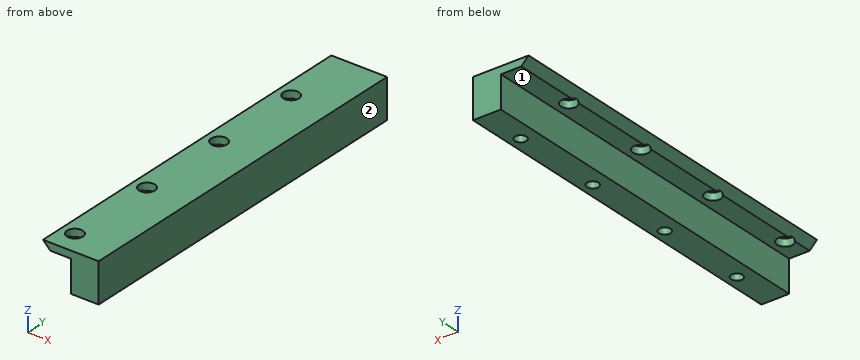
Autodesk Inventor part; units mm, degrees
ref_plane "Left_Connecting_Web_StartPlane" through (0, 0, 4) normal (0, 0, 1) x (1, 0, 0)
ref_plane "Left_Rod_Contact_Flange_StartPlane" through (0, 0, 10.9) normal (0, 0, 1) x (1, 0, 0)
ref_plane "Work Plane3" through (0, 0, 4) normal (0, 0, 1) x (1, 0, 0)
ref_plane "Left_Connecting_Web_StartPlane" through (0, 0, 4) normal (0, 0, 1) x (1, 0, 0)
sketch "Left_Connecting_Web_Profile" plane through (0, 0, 4) normal (0, 0, 1) x (1, 0, 0)
  line L0 (6, 0) -> (12, 0)
  line L1 (12, 0) -> (12, 80)
  line L2 (12, 80) -> (6, 80)
  line L3 (6, 80) -> (6, 0)
  point P0 (0, 0)
  dimension "d1" = 6
  dimension "d2" = 6
  dimension "d3" = 80
extrude "Left_Connecting_Web" add sketch "Left_Connecting_Web_Profile" along normal blind 8.5
ref_plane "Left_Rod_Contact_Flange_StartPlane" through (0, 0, 10.9) normal (0, 0, 1) x (1, 0, 0)
sketch "Left_Rod_Contact_Flange_Profile" plane through (0, 0, 10.9) normal (0, 0, 1) x (1, 0, 0)
  line L0 (0, 0) -> (12, 0)
  line L1 (12, 0) -> (12, 80)
  line L2 (12, 80) -> (0, 80)
  line L3 (0, 80) -> (0, 0)
  dimension "d7" = 12
  dimension "d8" = 80
extrude "Left_Rod_Contact_Flange" add sketch "Left_Rod_Contact_Flange_Profile" along normal blind 1.6
sketch "Original_Rod_Clearance_4x_Locations" plane through (0, 0, 0) normal (0, 0, 1) x (1, 0, 0)
  circle A0 centre (3, 5) radius 1.7
  circle A1 centre (3, 25) radius 1.7
  circle A2 centre (3, 45) radius 1.7
  circle A3 centre (3, 65) radius 1.7
  point P0 (0, 0)
  dimension "d11" = 3
  dimension "d12" = 5
  dimension "d13" = 3.4
  dimension "d14" = 3
  dimension "d15" = 25
  dimension "d16" = 3.4
  dimension "d17" = 3
  dimension "d18" = 45
  dimension "d19" = 3.4
  dimension "d20" = 3
  dimension "d21" = 65
  dimension "d22" = 3.4
extrude "Original_Rod_Clearance_4x" cut sketch "Original_Rod_Clearance_4x_Locations" along normal through all
ref_plane "Work Plane3" through (0, 0, 4) normal (0, 0, 1) x (1, 0, 0)
sketch "Deck_Assembly_M3_Locations" plane through (0, 0, 4) normal (0, 0, 1) x (1, 0, 0)
  circle A0 centre (9.5, 10) radius 1.25
  circle A1 centre (9.5, 30) radius 1.25
  circle A2 centre (9.5, 50) radius 1.25
  circle A3 centre (9.5, 70) radius 1.25
  point P0 (0, 0)
  dimension "d26" = 9.5
  dimension "d27" = 10
  dimension "d28" = 2.5
  dimension "d29" = 9.5
  dimension "d30" = 30
  dimension "d31" = 2.5
  dimension "d32" = 9.5
  dimension "d33" = 50
  dimension "d34" = 2.5
  dimension "d35" = 9.5
  dimension "d36" = 70
  dimension "d37" = 2.5
extrude "Four_Blind_M3_Tap_Bores" cut sketch "Deck_Assembly_M3_Locations" along normal blind 6.5
thread "Deck_M3x0_5_6H_1"
thread "Deck_M3x0_5_6H_2"
thread "Deck_M3x0_5_6H_3"
thread "Deck_M3x0_5_6H_4"
chamfer "Outer_End_1p6mm_45deg" distance 1.6 angle 45 1 edges at (0, 40, 10.9)
equation "\"d2\" = WebThickness"
equation "\"d3\" = ContactLength"
equation "\"d4\" = DropHeight"
equation "\"d7\" = RodWidth + WebThickness"
equation "\"d8\" = ContactLength"
equation "\"d9\" = RodFlangeThickness"
equation "\"d13\" = RodClearanceDiameter"
equation "\"d16\" = RodClearanceDiameter"
equation "\"d19\" = RodClearanceDiameter"
equation "\"d22\" = RodClearanceDiameter"
equation "\"d28\" = TapDrillDiameter"
equation "\"d31\" = TapDrillDiameter"
equation "\"d34\" = TapDrillDiameter"
equation "\"d37\" = TapDrillDiameter"
equation "\"d38\" = JoinThreadDepth"
equation "\"d40\" = JoinThreadDepth"
equation "\"d42\" = JoinThreadDepth"
equation "\"d44\" = JoinThreadDepth"
equation "\"d46\" = JoinThreadDepth"
equation "\"d48\" = OuterEndChamfer"
equation "\"d49\" = OuterEndChamfer"
equation "\"OverallWidth\" = 51"
equation "\"RodWidth\" = 6"
equation "\"ContactLength\" = 80"
equation "\"BaseThickness\" = 4"
equation "\"DropHeight\" = 8.5"
equation "\"WebThickness\" = 6"
equation "\"FingerStartX\" = 19.93338"
equation "\"FingerWidth\" = 13.5"
equation "\"FingerThickness\" = 6"
equation "\"FingerEndInset\" = 4"
equation "\"RodClearanceDiameter\" = 3.4"
equation "\"ClampFirstY\" = 41.82802"
equation "\"ClampPitch\" = 16"
equation "\"ClampHeight\" = BaseThickness + 0.5 * FingerThickness"
equation "\"TapDrillDiameter\" = 2.5"
equation "\"TapDepth\" = 6"
equation "\"RodHoleStart\" = 5"
equation "\"RodScrewPitch\" = 20"
equation "\"JoinLeftX\" = 9.5"
equation "\"JoinFirstY\" = 10"
equation "\"JoinPitch\" = 20"
equation "\"JoinThreadDepth\" = 6.5"
equation "\"JoinCountersinkDiameter\" = 6.2"
equation "\"d0\" = BaseThickness"
equation "\"d6\" = BaseThickness + DropHeight - RodFlangeThickness"
equation "\"d25\" = BaseThickness"
equation "\"RodFlangeThickness\" = 1.6"
equation "\"OuterEndChamfer\" = RodFlangeThickness"
properties part number "Left_Rod_Support"
Check sheet for the modelled part. Datum: model origin and axes. Units: mm. Face numbers are marked on the shaded views. A direction names the side the tool comes from. Round coordinates to 2 decimals unless told otherwise and drop trailing zeros. Loops run counter-clockwise (first coordinate to the right, second up) from the corner with the lowest first, then second, coordinate; pieces in that order, holes last. Notation, with made-up numbers: (62, 62.5) -> (109, 62.5) arc R33 ccw to (109, 96.5) -> close; hole circle Ø5 at (6, 15). An arc over 180 degrees is marked (long way). Answer in a Markdown table with one row per item.
Q1. Sectioned sample at D-D on x = 9.5. Enter the section's corners in (y, z).
Data:
| item | result |
|---|---|
| outline | (0, 4) -> (8.75, 4) -> (8.75, 10.5) -> (11.25, 10.5) -> (11.25, 4) -> (28.75, 4) -> (28.75, 10.5) -> (31.25, 10.5) -> (31.25, 4) -> (48.75, 4) -> (48.75, 10.5) -> (51.25, 10.5) -> (51.25, 4) -> (68.75, 4) -> (68.75, 10.5) -> (71.25, 10.5) -> (71.25, 4) -> (80, 4) -> (80, 12.5) -> (0, 12.5) -> close |
Q2. Set-up check for the marked faces 1 and 2: record each of +Z, -Z, +X, -X, +Y, -Y from which the full face is reachable in a straight line by a thin tool's end or side.
Data:
| item | result |
|---|---|
| face 1 | -Z, -X, +Y, -Y |
| face 2 | +Z, -Z, +X, +Y, -Y |
Q3. Thickness scan on L1, parallel to Y at x = 9.5, z = 5.75; L2, parallel to Y at x = 3, z = 11.6; L3, parallel to X at y = 19, z = 8.25. Record the ranges inside material, lowest first.
Data:
| item | result |
|---|---|
| L1 | y = 0 to 8.75, 11.25 to 28.75, 31.25 to 48.75, 51.25 to 68.75, 71.25 to 80 |
| L2 | y = 0 to 3.3, 6.7 to 23.3, 26.7 to 43.3, 46.7 to 63.3, 66.7 to 80 |
| L3 | x = 6 to 12 |
Q4. Sectioned sample at B-B on z = 5.25. Enter the section's corners in (x, y), then the cut area to 3 significant figures.
Data:
| item | result |
|---|---|
| outline | (6, 0) -> (12, 0) -> (12, 80) -> (6, 80) -> close; hole circle Ø2.5 at (9.5, 10); hole circle Ø2.5 at (9.5, 30); hole circle Ø2.5 at (9.5, 50); hole circle Ø2.5 at (9.5, 70) |
| area | 460 mm^2 |
Q5. Sectioned sample at A-A on y = 65. Enter the section's corners in (x, z), then the cut area to 3 significant figures.
Data:
| item | result |
|---|---|
| outline | (0, 12.5) -> (1.3, 11.2) -> (1.3, 12.5) -> close; (4.7, 10.9) -> (6, 10.9) -> (6, 4) -> (12, 4) -> (12, 12.5) -> (4.7, 12.5) -> close |
| area | 53.9 mm^2 |
Q6. Sectioned sample at C-C on y = 30. Enter the section's corners in (x, z), then the cut area to 3 significant figures.
Data:
| item | result |
|---|---|
| outline | (0, 12.5) -> (1.6, 10.9) -> (6, 10.9) -> (6, 4) -> (8.25, 4) -> (8.25, 10.5) -> (10.75, 10.5) -> (10.75, 4) -> (12, 4) -> (12, 12.5) -> close |
| area | 43.1 mm^2 |
Q7. Go/stop test with flat-tipped pins: P1, Ø2, axis at x = 3, y = 65, coming from the +Z side; P2, Ø1.2, axis at x = 9.5, y = 50, coming from the -Z side; P3, Ø1, axis at y = 33, z = 8.5, coming from the -X side. Record where each tip stops, or that it passes through.
Data:
| item | result |
|---|---|
| P1 | passes through |
| P2 | stops at z = 10.5 |
| P3 | stops at x = 6 |
